Geometry: final body of the model. Coordinates: model frame, mm. Face numbers are marked on the shaded views. Coordinates: 2 decimals unless noted, no trailing zeros. Write each loop counter-clockwise with the first axis right and the second up, starting at its lowest first coordinate (ties: lowest second). Pieces come first, ordered by that corner, then holes. Notation, with made-up numbers: (36.5, 85) -> (56.5, 85) arc R14 cw to (56.5, 95) -> close; hole circle Ø7 at (0, -26.5). An arc over 180 degrees is marked (long way). Answer as a JSON object with one key per item and string values. Group by question number.
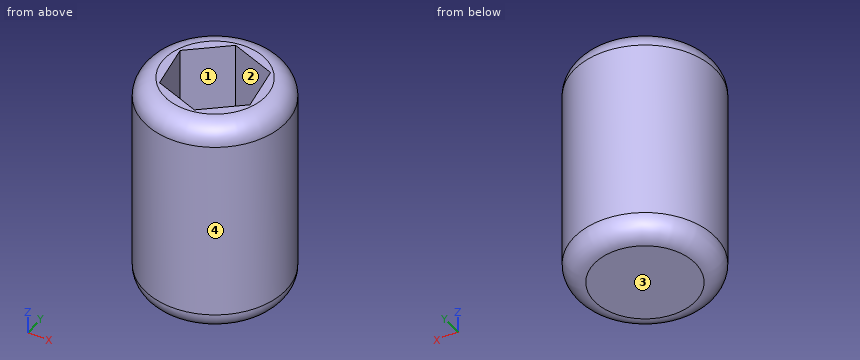
```python
from build123d import *

# Parameters (mm, degrees)
F0_R     = 44.45
F1_DEPTH = 139.7
F2_R     = 12.7
F3_R     = 22.915051
F4_DEPTH = 127
F6_DEPTH = 127


with BuildPart() as f1:
    # F0 (on Top) → F1 (new body)
    with BuildSketch(Plane.XY):
        Circle(F0_R)
    extrude(amount=F1_DEPTH)

    # F2
    f2_edges = [f1.edges().sort_by_distance(p)[0] for p in [
        (-44.45, 0, 0),
        (-44.45, 0, 139.7),
    ]]
    fillet(f2_edges, radius=F2_R)

    # F3 (on face) → F4 (cut)
    with BuildSketch(Plane.XY.offset(139.7)):
        Circle(F3_R)
    extrude(amount=-F4_DEPTH, mode=Mode.SUBTRACT)

    # F5 (on face) → F6 (cut)
    with BuildSketch(Plane.XY.offset(139.7)):
        Polygon((28.460228, -9.844098), (22.755353, 19.725232), (-5.704875, 29.56933), (-28.460228, 9.844098), (-22.755353, -19.725232), (5.704875, -29.56933), align=None)
    extrude(amount=-F6_DEPTH, mode=Mode.SUBTRACT)


solid = f1.part
```
Item 1: Section A-A on z = 108. Output: boundary loops of the cut face in (x, y), then the cut area to 3 significant figures.
Item 2: Ray query, L1, parallel to Z at x = -16, y = -18; L2, parallel to Y at x = 14.5, z = 99.5; L3, parallel to Y at x = -0.5, z = 52. Return the intervals inside material, ascending. Write a range as [from, to].
Item 3: Section C-C on y = 0. Output: boundary loops of the cut face in (x, z), then the cut area to 3 significant figures.
Item 4: Contact query for flat-ended pins moving along their axis: pin 1 (1.5 mm diameter, centred on x = 1, y = 1.5, fed in from +Z); pin 2 (4 mm diameter, centred on x = -26.5, y = 31, fed in from -Z); pin 3 (1 mm diameter, centred on x = 27.5, z = 115.5, fed in from -Y). Output: stop coordinate, or through.
Item 5: Section B-B on x = 0. Output: boundary loops of the cut face in (y, z).
Item 6: Mould query, pull axis X, two halves, no side actions, for the marked faces 1, 2, 3 and 4. Classes: +X half, -X half, draft (parallel to the pull), parting line (faces both ways), or undercut.
Answer sheet:
{
 "1": {"outline": "circle Ø88.9 at (0, 0); hole (-28.46, 9.84) -> (-22.76, -19.73) -> (5.7, -29.57) -> (28.46, -9.84) -> (22.76, 19.73) -> (-5.7, 29.57) -> close", "area": "3,850 mm^2"},
 "2": {"L1": "z = [0, 12.7]", "L2": "y = [-42.02, -21.95], [22.58, 42.02]", "L3": "y = [-44.45, -27.42], [27.77, 44.45]"},
 "3": {"outline": "(-44.45, 12.7) arc R12.7 ccw to (-31.75, 0) -> (31.75, 0) arc R12.7 ccw to (44.45, 12.7) -> (44.45, 127) arc R12.7 ccw to (31.75, 139.7) -> (26.56, 139.7) -> (26.56, 12.7) -> (-26.56, 12.7) -> (-26.56, 139.7) -> (-31.75, 139.7) arc R12.7 ccw to (-44.45, 127) -> close", "area": "5,530 mm^2"},
 "4": {"pin 1": "stops at z = 12.7", "pin 2": "stops at z = 2.13", "pin 3": "stops at y = -35.31"},
 "5": {"outline": "(-44.45, 12.7) arc R12.7 ccw to (-31.75, 0) -> (31.75, 0) arc R12.7 ccw to (44.45, 12.7) -> (44.45, 127) arc R12.7 ccw to (31.75, 139.7) -> (27.6, 139.7) -> (27.6, 12.7) -> (-27.6, 12.7) -> (-27.6, 139.7) -> (-31.75, 139.7) arc R12.7 ccw to (-44.45, 127) -> close"},
 "6": {"face 1": "undercut", "face 2": "undercut", "face 3": "draft", "face 4": "parting line"}
}
